For this review, use the dimensioned drawing (mm, ordinates from the lowest corner) and the shaded views. A direction names the side the tool comes from. Give positions to 0.01 mm unless a question says otherwise; leave off trailing zeros. Loops run counter-clockwise (first coordinate to the right, second up) from the corner with the lowest first, then second, coordinate; pieces in that order, holes last. Notation, with made-up numbers: (76.25, 65) - (92.25, 65) arc R21 cw to (92.25, 72) - close; hole circle Ø5 at (0, 12.5). An arc over 180 degrees is marked (long way). Put each result on its own line as item: value.
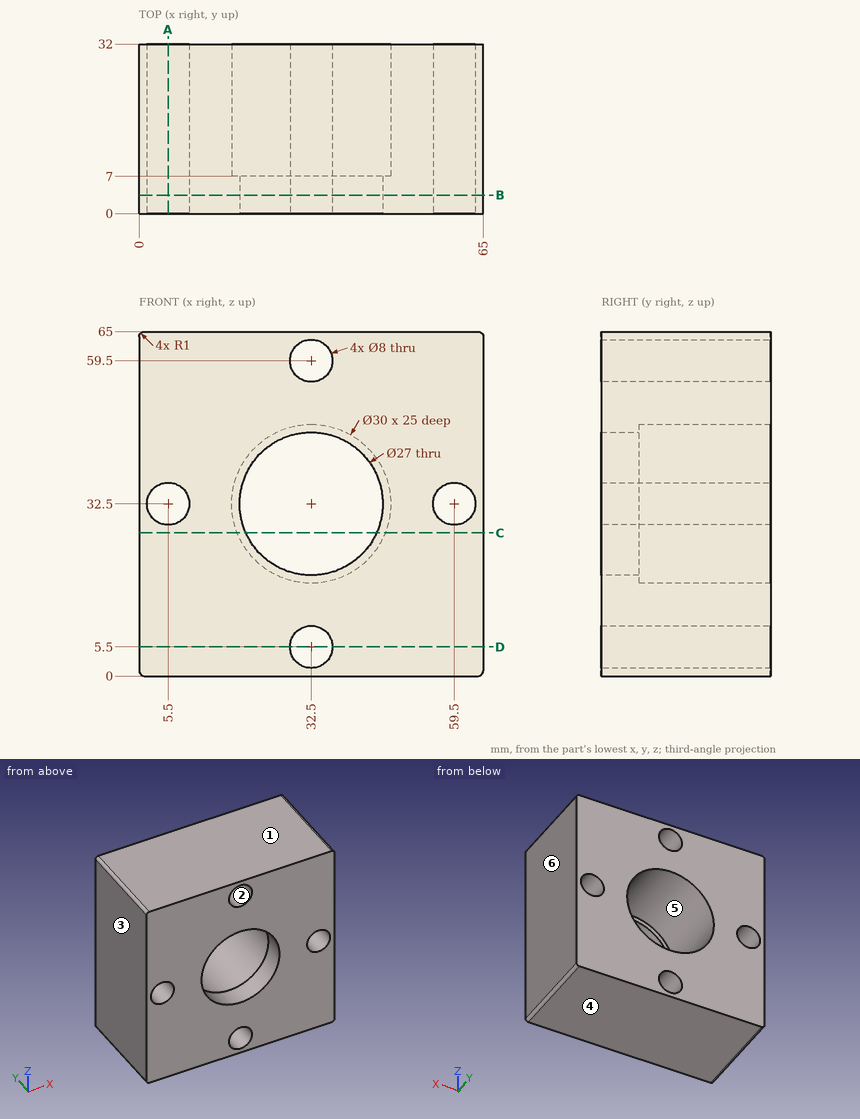
1) Wall thickness on line 1 (X direction, y = 13, z = 32.5); line 2 (X direction, y = 23, z = 34); line 3 (Z direction, x = 32, y = 24): over which ranges is each line inside the solid? List them lowest first.
Geometry check:
line 1: x = 0 to 1.5, 9.5 to 17.5, 47.5 to 55.5, 63.5 to 65
line 2: x = 0 to 1.79, 9.21 to 17.58, 47.42 to 55.79, 63.21 to 65
line 3: z = 0 to 1.53, 9.47 to 17.51, 47.49 to 55.53, 63.47 to 65
2) Take a section at A-A on x = 5.5. State the section outline as (y, z) points.
Geometry check:
outline: (0, 0) - (32, 0) - (32, 28.5) - (0, 28.5) - close; (0, 36.5) - (32, 36.5) - (32, 65) - (0, 65) - close
3) Take a section at B-B on y = 3.5. State the section outline as (x, z) points, and give its area (3 significant figures).
Geometry check:
outline: (0, 1) arc R1 ccw to (1, 0) - (64, 0) arc R1 ccw to (65, 1) - (65, 64) arc R1 ccw to (64, 65) - (1, 65) arc R1 ccw to (0, 64) - close; hole circle Ø8 at (5.5, 32.5); hole circle Ø27 at (32.5, 32.5); hole circle Ø8 at (32.5, 5.5); hole circle Ø8 at (32.5, 59.5); hole circle Ø8 at (59.5, 32.5)
area: 3,450 mm²
4) Draft analysis for pull direction Z (two halves, no side actions). For the marked faces 1, 2, 3 and 4, state which applies: pulls with the +Z half, pulls with the -Z half, needs draft (parallel to the pull), parting line crosses it, or undercut.
Geometry check:
face 1: pulls with the +Z half
face 2: undercut
face 3: needs draft
face 4: pulls with the -Z half
5) For the marked faces 5 and 6, list the 3-axis set-ups (+Z, -Z, +X, -X, +Y, -Y) from which the entire face can be reached by the end or side of a thin tool; tool diameter is ignored.
Geometry check:
face 5: +Y
face 6: +Z, -Z, +X, +Y, -Y
6) Insertion check: pin 1 Ø15 at (x, z) = (39, 31) entering from +Y. The pin has a flat end and moves straight along its axis. Give the tip position at first contact, or say it passes through.
Geometry check:
pin 1: stops at y = 7
7) Take a section at D-D on z = 5.5. State the section outline as (x, y) points.
Geometry check:
outline: (0, 0) - (28.5, 0) - (28.5, 32) - (0, 32) - close; (36.5, 0) - (65, 0) - (65, 32) - (36.5, 32) - close
8) Take a section at C-C on z = 27. State the section outline as (x, y) points.
Geometry check:
outline: (0, 0) - (20.17, 0) - (20.17, 7) - (18.54, 7) - (18.54, 32) - (0, 32) - close; (44.83, 0) - (65, 0) - (65, 32) - (46.46, 32) - (46.46, 7) - (44.83, 7) - close
